Verification items for the finished model (mm, model axes). A direction names the side the tool comes from. Coordinates: 2 decimals unless noted, no trailing zeros. Loops run counter-clockwise (first coordinate to the right, second up) from the corner with the lowest first, then second, coordinate; pieces in that order, holes last. Notation, with made-up numbers: M 37,40.25 L 68,40.25 A28 ccw 68,75.25 Z; hole C 30.25,87.25 d10. An arc over 180 degrees is marked long. Write item = value, one per line. Start each with the question number.
```python
from build123d import *

# Parameters (mm, degrees)
BOSS_EXTRUDE1_DEPTH            = 10
HOLE1_D                        = 6.35
HOLE1_DEPTH                    = 2
F_25_0_25_DIAMETER_HOLE1_D     = 25
F_25_0_25_DIAMETER_HOLE1_DEPTH = 10
SCALE1_SCALE                   = 4


with BuildPart() as part:
    # Sketch1 → Boss-Extrude1 (new body)
    with BuildSketch(Plane.XZ.offset(10)):
        with BuildLine():
            Line((55, 0), (-55, 0))
            Line((-55, 0), (-55, -2))
            Line((-55, -2), (-14.361406616, -2))
            ThreePointArc((-14.361406616, -2), (0, -14.5), (14.361406616, -2))
            Line((14.361406616, -2), (55, -2))
            Line((55, -2), (55, 0))
        make_face()
    extrude(amount=-BOSS_EXTRUDE1_DEPTH)

    # Hole1
    with Locations(Plane(origin=(0, 0, -2), x_dir=(-1, 0, 0), z_dir=(0, 0, -1))):
        with Locations((-50, -5), (50, -5)):
            Hole(HOLE1_D / 2, depth=HOLE1_DEPTH)

    # Ø25.0 (25) Diameter Hole1
    with Locations(Plane(origin=(0, -10, 0), x_dir=(-1, 0, 0), z_dir=(0, -1, 0))):
        with Locations((0, 0)):
            Hole(F_25_0_25_DIAMETER_HOLE1_D / 2, depth=F_25_0_25_DIAMETER_HOLE1_DEPTH)


with BuildPart() as part_1:
    # Scale1: scaled about (0, -5, -3.754985593)
    add(part.part.scale(SCALE1_SCALE).moved(Location((0, 15, 11.264956779))))


solid = part_1.part
```
Q1. Sectioned sample at C-C on z = -11. Record the cut outline in (x, y), plus the area to 3 significant figures.
Q2. Mould release check, pull along X, two halves, no side actions. Record for faces 1 (the face through (1.099, -4.72, -38.723)), 2 (the face through (-220, -5, 7)), 3 (the face through (-1.163, -5.28, -46.723)), 4 (the face through (-140, -5, 3.265)): +X half, -X half, draft (parallel to the pull), parting line (faces both ways), or undercut.
Q3. Sectioned sample at D-D on x = -80. Record the cut outline in (y, z).
Q4. Scan lines: L1, parallel to Y at x = -200, z = 8.75; L2, parallel to Z at x = 78, y = -16; L3, parallel to X at y = -4.5, z = -27.5. Record each from-to range of solid material in increasing order. Write a range as [from, to].
Q5. Gauge pin test, flat ends, axial feed: pin 1 (12 mm diameter, centred on x = 41, z = -14, fed in from -Y); pin 2 (5 mm diameter, centred on x = -49.5, z = -25, fed in from +Y); pin 3 (2 mm diameter, centred on x = -175, y = -15, fed in from -Z); pin 4 (4 mm diameter, centred on y = -18, z = -11.5, fed in from +X). Record the tip position at first contact, or that the pin passes through.
Q6. Set-up check for faces 5 (the face through (138, -5, 3.265)), 6 (the face through (220, -5, 7)): record each of +Z, -Z, +X, -X, +Y, -Y from which the full face is reachable in a straight line by a thin tool's end or side.
Q7. Sectioned sample at B-B on y = -5. Record the cut outline in (x, z).
Q8. Sectioned sample at A-A on x = 200. Record the cut outline in (y, z).
Solutions:
q1.outline = M -53.56,-25 L -44.77,-25 L -44.77,15 L -53.56,15 Z; M 44.77,-25 L 53.56,-25 L 53.56,15 L 44.77,15 Z
q1.area = 703 mm²
q2.face_1 = undercut
q2.face_2 = -X half
q2.face_3 = parting line
q2.face_4 = draft
q3.outline = M -25,3.26 L 15,3.26 L 15,11.26 L -25,11.26 Z
q4.L1 = [-25, -17.7], [7.7, 15]
q4.L2 = [3.26, 11.26]
q4.L3 = [-43.14, -31.58], [31.58, 43.14]
q5.pin_1 = -25
q5.pin_2 = through
q5.pin_3 = 3.26
q5.pin_4 = 54.16
q6.face_5 = -Z, +X, +Y, -Y
q6.face_6 = +Z, -Z, +X, +Y, -Y
q7.outline = M -220,3.26 L -212.7,3.26 L -212.7,11.26 L -220,11.26 Z; M -187.3,3.26 L -57.45,3.26 A58 ccw 57.45,3.26 L 187.3,3.26 L 187.3,11.26 L 50,11.26 A50 cw -50,11.26 L -187.3,11.26 Z; M 212.7,3.26 L 220,3.26 L 220,11.26 L 212.7,11.26 Z
q8.outline = M -25,3.26 L -17.7,3.26 L -17.7,11.26 L -25,11.26 Z; M 7.7,3.26 L 15,3.26 L 15,11.26 L 7.7,11.26 Z
